Design review of the part built by this model. Coordinates are the model's own, in mm. Coordinates: 2 decimals unless noted, no trailing zeros. Loops run counter-clockwise (first coordinate to the right, second up) from the corner with the lowest first, then second, coordinate; pieces in that order, holes last. Notation, with made-up numbers: (-4.5, 51.25) -> (54.5, 51.25) arc R20 ccw to (54.5, 83.25) -> close; hole circle Ø3 at (76, 51.5). An arc over 180 degrees is marked (long way). Answer in a Markdown table with one row per item.
Autodesk Inventor part; units mm, degrees
ref_plane "Work Plane4" through (60.2613, -49.3334, 0) normal (0, 1, 0) x (1, 0, 0)
ref_plane "YZ Plane" through (0, 0, 0) normal (1, 0, 0) x (0, 1, 0)
ref_plane "XZ Plane" through (0, 0, 0) normal (0, 1, 0) x (-1, 0, 0)
ref_plane "Work Plane4" through (60.2613, -49.3334, 0) normal (0, 1, 0) x (1, 0, 0)
sketch "dimensions" plane through (60.2613, -49.3334, 0) normal (0, 1, 0) x (1, 0, 0)
  line L0 (-254, 127) -> (254, 127)
  line L1 (254, 127) -> (254, -127)
  line L2 (254, -127) -> (-254, -127)
  line L3 (-254, -127) -> (-254, 127)
  line L4 (-254, 127) -> (254, -127) construction
  line L5 (254, 127) -> (-254, -127) construction
  line L6 (-254, 0) -> (254, 0) construction
  circle A0 centre (177.8, 0) radius 10.5
  circle A1 centre (177.8, 0) radius 47.15 construction
  circle A2 centre (-203.2, 0) radius 9.5
  circle A3 centre (-203.2, 0) radius 23.9 construction
  circle A4 centre (2.7586, -32.2833) radius 2.1
  circle A5 centre (28.0468, -16.173) radius 2.1
  circle A6 centre (28.0468, 16.2948) radius 2.1
  circle A7 centre (-0.0711, 32.5287) radius 2.1
  circle A8 centre (-28.1891, 16.2948) radius 2.1
  circle A9 centre (-28.1891, -16.173) radius 2.1
  circle A10 centre (-0.0711, 0.0609) radius 6.35
  line L7 (177.8, 0) -> (-203.2, 0) construction
  circle A11 centre (76.2, 0) radius 5
  circle A12 centre (-101.6, 0) radius 5
  dimension "d1" = 508
  dimension "d2" = 254
  dimension "d3" = 21
  dimension "d4" = 94.3
  dimension "d6" = 19
  dimension "d7" = 47.8
  dimension "d32" = 10
  dimension "d34" = 101.6
  dimension "d35" = 10
  dimension "d36" = 101.6
extrude "Extrusion5" add sketch "dimensions" along normal blind 5 contours L0 L1 L2 L3 | A11 | A12
fillet "Fillet6" radius 12.7 4 edges at (314.2613, -46.8334, -127) (-193.7387, -46.8334, -127) (-193.7387, -46.8334, 127) (314.2613, -46.8334, 127)
extrude "Extrusion6" cut sketch "dimensions" along normal up to next contours A11 | A12
equation "\"d37\" = d36"
properties part number "antenna-mount"
(1) Draft analysis for pull direction X (two halves, no side actions). For faces 1 (the cylindrical face through (310.64, -46.8, -123.18)), 2 (the cylindrical face through (-36.72, -46.87, -1.92)), 3 (the flat face through (57, -44.333, -30)), state which applies: pulls with the +X half, pulls with the -X half, needs draft (parallel to the pull), parting line crosses it, or undercut.
Evaluation:
| item | result |
|---|---|
| face 1 | pulls with the +X half |
| face 2 | undercut |
| face 3 | needs draft |
(2) For pin 1 (11.5 mm diameter, centred on x = -142.94, z = 0, fed in from +Y), flat-tipped, find the tip position at first contact; note if it passes through.
Evaluation:
| item | result |
|---|---|
| pin 1 | passes through |
(3) To check wall thickness, follow probe 1 along X at (y, z) = (-45.9, 0); probe 2 along X at (y, z) = (-46.8, -14.5); probe 3 along X at (y, z) = (-45.55, 115). State the ranges of each line that lie inside material, in increasing order.
Evaluation:
| item | result |
|---|---|
| probe 1 | x = -193.74 to -152.44, -133.44 to -46.34, -36.34 to 53.84, 66.54 to 131.46, 141.46 to 227.56, 248.56 to 314.26 |
| probe 2 | x = -193.74 to 30.98, 33.16 to 87.22, 89.4 to 314.26 |
| probe 3 | x = -193.72 to 314.24 |
(4) Take a section at A-A on x = -145.5. Give the boundary of the cut face in (y, z), and give its area (3 significant figures).
Evaluation:
| item | result |
|---|---|
| outline | (-49.33, -127) -> (-44.33, -127) -> (-44.33, -9.15) -> (-49.33, -9.15) -> close; (-49.33, 9.15) -> (-44.33, 9.15) -> (-44.33, 127) -> (-49.33, 127) -> close |
| area | 1,180 mm² |
